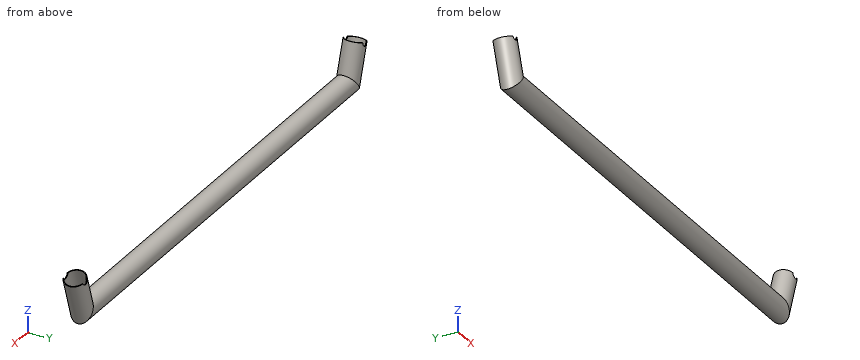
```python
from build123d import *

# Parameters (mm, degrees)
SKETCH2_R               = 10.5
SKETCH2_R_2             = 9.75
CUT_EXTRUDE1_DEPTH      = 255.202518271
CUT_EXTRUDE1_DEPTH_BACK = 255.202518271
SKETCH3_R               = 3.5


with BuildPart() as part:
    # Sweep1: sweep along a path in Sketch1
    with BuildLine(Plane(origin=(0, 0, 0), x_dir=(1, 0, 0), z_dir=(0, 1, 0))) as sweep1_path:
        Line((-240.81, -36.88), (-228.826961603, 0))
        Line((-228.826961603, 0), (228.826961603, 0))
        Line((228.826961603, 0), (240.81, -36.88))
    # Sketch2 → Sweep1 (sweep)
    with BuildSketch(Plane(origin=(-240.81, 0, 36.88), x_dir=(0.9510565162951523, 0, 0.3090169943749515), z_dir=(-0.3090169943749515, 0, 0.9510565162951523))):
        Circle(SKETCH2_R)
        Circle(SKETCH2_R_2, mode=Mode.SUBTRACT)
    sweep(path=sweep1_path.line, transition=Transition.RIGHT)

    # Sketch3 → Cut-Extrude1 (cut, two sides: drawn at the far end of the back side and taken through both)
    with BuildSketch(Plane(origin=(0, 0, 0), x_dir=(1, 0, 0), z_dir=(0, 1, 0)).offset(-CUT_EXTRUDE1_DEPTH_BACK)):
        with Locations((240.81, -36.88)):
            Circle(SKETCH3_R)
        with Locations((-240.81, -36.88)):
            Circle(SKETCH3_R)
    extrude(amount=CUT_EXTRUDE1_DEPTH + CUT_EXTRUDE1_DEPTH_BACK, mode=Mode.SUBTRACT)


solid = part.part
```
Geometry check sheet. Reference: the model listing, model coordinates, mm. Round coordinates to 2 decimals unless told otherwise and drop trailing zeros. Loops run counter-clockwise (first coordinate to the right, second up) from the corner with the lowest first, then second, coordinate; pieces in that order, holes last. Notation, with made-up numbers: M 25.5,58 L 83.5,58 A14 cw 83.5,78 Z; hole C 65.5,88 d5. An arc over 180 degrees is marked long. Return JSON: item names as keys, results as strings. Group by question number.
(1) Section check B-B, the plane x = -145.5. Enter the section's corners in (y, z), and give its area (3 significant figures).
(2) Go/stop test with flat-tipped pins: pin 1 (6 mm diameter, centred on x = -80.5, z = 9, fed in from +Y); pin 2 (8 mm diameter, centred on y = -1, z = 23, fed in from -X); pin 3 (4 mm diameter, centred on y = 5, z = 1.5, fed in from +X). Record where each tip stops, or that it passes through.
(3) Section check C-C, the plane z = 23. Give the number of separate pieces and of enclosed holes in the cut face, and give its area (3 significant figures).
(4) Scan lines: line 1 along X through (y, z) = (5.5, 24); line 2 along X through (y, z) = (-6.75, 32); line 3 along X through (y, z) = (4.5, 37). Record each from-to range of solid material in increasing order. Write a range as [from, to].
(5) Section check A-A, the plane y = 0. Enter the section's corners in (x, z).
Data:
{
 "1": {"outline": "C 0,0 d21; hole C 0,0 d19.5", "area": "47.7 mm²"},
 "2": {"pin 1": "y = 8.62", "pin 2": "x = -248.62", "pin 3": "x = 240.15"},
 "3": {"separate pieces": "2", "enclosed holes": "2", "area": "100 mm²"},
 "4": {"line 1": "[-246.03, -245.09], [-228.16, -227.22], [227.22, 228.16], [245.09, 246.03]", "line 2": "[-247.68, -246.62], [-231.83, -230.77], [230.77, 231.83], [246.62, 247.68]", "line 3": "[-231.75, -230.87], [230.87, 231.75]"},
 "5": {"outline": "M -250.8,33.64 L -236.46,-10.5 L 236.46,-10.5 L 250.8,33.64 L 250.08,33.87 L 235.91,-9.75 L -235.91,-9.75 L -250.08,33.87 Z; M -231.54,39.89 L -221.74,9.75 L 221.74,9.75 L 231.54,39.89 L 230.82,40.12 L 221.2,10.5 L -221.2,10.5 L -230.82,40.12 Z"}
}
